Part model, mm, in its own coordinate system. A direction names the side the tool comes from. Give positions to 0.01 mm unless a question says otherwise; leave off trailing zeros. Order: outer loops, then holes, each group sorted by start corner. A loop starts at its lowest first (then second) coordinate and runs counter-clockwise, first axis right, second up.
from build123d import *

# Parameters (mm, degrees)
SKETCH1_R           = 3
BOSS_EXTRUDE1_DEPTH = 3.175
BOSS_EXTRUDE2_DEPTH = 3.175


with BuildPart() as part:
    # Sketch1 → Boss-Extrude1 (new body)
    with BuildSketch(Plane.XY):
        Polygon((15, 60), (0, 45), (0, 0), (30, 0), (30, 60), align=None)
        with Locations((15, 15)):
            Circle(SKETCH1_R, mode=Mode.SUBTRACT)
    extrude(amount=BOSS_EXTRUDE1_DEPTH)

    # Sketch2 → Boss-Extrude2 (add)
    with BuildSketch(Plane.XY.offset(3.175)):
        Polygon((15, 60), (0, 45), (0, 35), (30, 35), (30, 45), (30, 60), align=None)
    extrude(amount=BOSS_EXTRUDE2_DEPTH)


solid = part.part
Item 1: Band-saw the part on B-B on z = 1. List the corners of the cut face in (x, y), plus the area to 3 significant figures.
Item 2: Band-saw the part on D-D on z = 5.25. List the corners of the cut face in (x, y), plus the area to 4 significant figures.
Item 3: Which spindle directions (+Z, -Z, +X, -X, +Y, -Y) get a long thin tool onto all of the face, cutting with end or side? Do faces 5 (the face through (15, 0, 2)), 6 (the face through (11, 18, 3.175)). Say none if no direction does.
Item 4: Band-saw the part on A-A on y = 15. List the corners of the cut face in (x, z) (3 decimals), plus the area to 3 significant figures.
Item 5: Band-saw the part on C-C on x = 6.25. List the corners of the cut face in (y, z) (3 decimals), plus the area to 3 significant figures.
Item 6: Drop flat-ended pins along their axis: P1, Ø15, axis at x = 15, y = 12, coming from the +Z side (3 decimals); P2, Ø3.5, axis at x = 15, y = 15, coming from the +Z side; P3, Ø2, axis at x = 3.5, z = 4.5, coming from the -Y side. Give the stop position or say it passes through.
Item 7: Pull direction X, two halves, no side cores. Call faces 1 (the face through (18, 48, 6.35)), 2 (the face through (8, 53, 3)), 3 (the face through (30, 36, 2)), 4 (the face through (12.6, 13.2, 1.6)): released by +X, released by -X, zero draft, split by the parting line, or undercut.
Item 8: Drill centre lines: probe 1 along Y at (x, z) = (15, 2.2); probe 2 along Z at (x, y) = (17.5, 10) (3 decimals); probe 3 along Y at (x, z) = (25, 4.5). Where is each one in solid material? Low to high.
Working result:
1. outline: (0, 0) - (30, 0) - (30, 60) - (15, 60) - (0, 45) - close; hole circle Ø6 at (15, 15)
1. area: 1,660 mm2
2. outline: (0, 35) - (30, 35) - (30, 60) - (15, 60) - (0, 45) - close
2. area: 637.5 mm2
3. face 5: +Z, -Z, +X, -X, -Y
3. face 6: +Z, +X, -X, -Y
4. outline: (0, 0) - (12, 0) - (12, 3.175) - (0, 3.175) - close; (18, 0) - (30, 0) - (30, 3.175) - (18, 3.175) - close
4. area: 76.2 mm2
5. outline: (0, 0) - (51.25, 0) - (51.25, 6.35) - (35, 6.35) - (35, 3.175) - (0, 3.175) - close
5. area: 214 mm2
6. P1: stops at z = 3.175
6. P2: passes through
6. P3: stops at y = 35
7. face 1: zero draft
7. face 2: released by -X
7. face 3: released by +X
7. face 4: undercut
8. probe 1: y = 0 to 12, 18 to 60
8. probe 2: z = 0 to 3.175
8. probe 3: y = 35 to 60
